Check sheet for the modelled part. Datum: model origin and axes. Units: mm. Round coordinates to 2 decimals unless told otherwise and drop trailing zeros. Loops run counter-clockwise (first coordinate to the right, second up) from the corner with the lowest first, then second, coordinate; pieces in that order, holes last. Notation, with made-up numbers: (38.25, -20) -> (85.25, -20) arc R21 ccw to (85.25, 6) -> close; hole circle Ø7 at (39.25, 5). An arc over 180 degrees is marked (long way). Return JSON: item names as keys, results as strings.
from build123d import *

# Parameters (mm, degrees)
SKETCH_1_W      = 130
SKETCH_1_H      = 40
SKETCH_1_R      = 8.5
EXTRUDE_1_DEPTH = 8
CHAMFER_1_SIZE  = 5


with BuildPart() as part:
    # 草图1 → 凸台-拉伸1 (new body)
    with BuildSketch(Plane(origin=(0, 0, 0), x_dir=(1, 0, 0), z_dir=(0, 1, 0))):
        with Locations((65, 20)):
            Rectangle(SKETCH_1_W, SKETCH_1_H)
        with Locations(Location((20, 20, 0), (0, 0, 270))):
            Circle(SKETCH_1_R, mode=Mode.SUBTRACT)
        with Locations(Location((110, 20, 0), (0, 0, 270))):
            Circle(SKETCH_1_R, mode=Mode.SUBTRACT)
    extrude(amount=EXTRUDE_1_DEPTH)

    # 倒角1
    chamfer_1_edges = [part.edges().sort_by_distance(p)[0] for p in [
        (0, 4, -40),
        (130, 4, -40),
        (130, 4, 0),
        (0, 4, 0),
    ]]
    chamfer(chamfer_1_edges, length=CHAMFER_1_SIZE)


solid = part.part
Q1. Section check A-A (z = -24). Record the boundary of the cut face in (x, y), then the cut area to 3 significant figures.
Results list:
{"outline": "(0, 0) -> (12.5, 0) -> (12.5, 8) -> (0, 8) -> close; (27.5, 0) -> (102.5, 0) -> (102.5, 8) -> (27.5, 8) -> close; (117.5, 0) -> (130, 0) -> (130, 8) -> (117.5, 8) -> close", "area": "800 mm^2"}
Q2. Material ranges on line 1 (X direction, y = 2, z = -20); line 2 (X direction, y = 3.5, z = -16); line 3 (Z direction, x = 17, y = 5), recorded low to high.
Results list:
{"line 1": "0 to 11.5, 28.5 to 101.5, 118.5 to 130", "line 2": "0 to 12.5, 27.5 to 102.5, 117.5 to 130", "line 3": "-40 to -27.95, -12.05 to 0"}
Q3. Section check D-D (z = -2.5). Record the boundary of the cut face in (x, y).
Results list:
{"outline": "(2.5, 0) -> (127.5, 0) -> (127.5, 8) -> (2.5, 8) -> close"}
Q4. Go/stop test with a flat-tipped pin: pin 1 (13.5 mm diameter, centred on x = 110, z = -20, fed in from -Y). Record where the tip stops, or that it passes through.
Results list:
{"pin 1": "through"}
Q5. Section check C-C (x = 110). Record the boundary of the cut face in (y, z), then the cut area to 3 significant figures.
Results list:
{"outline": "(0, -40) -> (8, -40) -> (8, -28.5) -> (0, -28.5) -> close; (0, -11.5) -> (8, -11.5) -> (8, 0) -> (0, 0) -> close", "area": "184 mm^2"}
Q6. Draft check along X on faces 1 (the flat face through (64, 4, -40)), 2 (the cylindrical face through (11.7, 3.94, -21.84)), 3 (the flat face through (130, 4, -20)), 4 (the flat face through (0, 4, -20)). Enter one of: released by +X, released by -X, zero draft, split by the parting line, or undercut.
Results list:
{"face 1": "zero draft", "face 2": "undercut", "face 3": "released by +X", "face 4": "released by -X"}
Q7. Section check B-B (y = 5). Record the boundary of the cut face in (x, z).
Results list:
{"outline": "(0, -35) -> (5, -40) -> (125, -40) -> (130, -35) -> (130, -5) -> (125, 0) -> (5, 0) -> (0, -5) -> close; hole circle Ø17 at (20, -20); hole circle Ø17 at (110, -20)"}
